The figure shows three views and two pictorial views of one solid part (mm, origin at its lowest corner). Answer the questions. A direction names the side the tool comes from. Coordinates: 2 decimals unless noted, no trailing zeros. Loops run counter-clockwise (first coordinate to the right, second up) from the corner with the lowest first, then second, coordinate; pieces in that order, holes last. Notation, with made-up numbers: (-39, -40) - (15, -40) arc R22 cw to (15, -33) - close; hole circle Ø4 at (33.25, 3.5). An arc over 180 degrees is marked (long way). One line per question, with ' | ' between items.
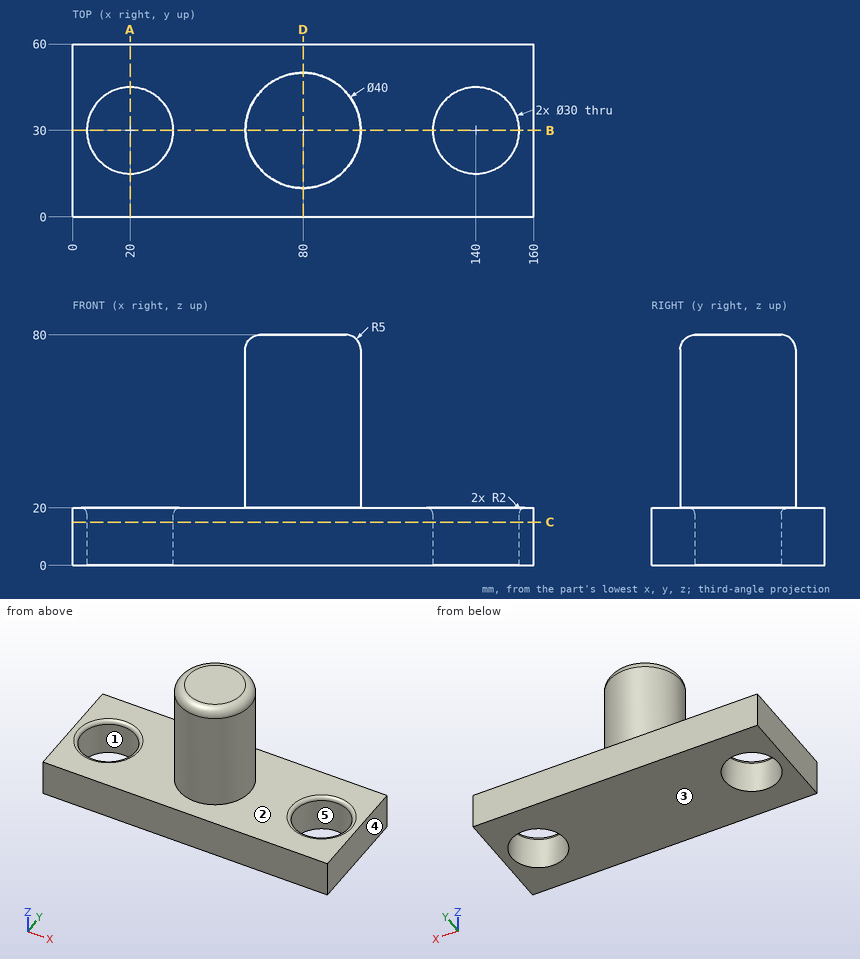
Item 1: Find the intervals of material crossed by line 1 (Y direction, x = 20, z = 8); line 2 (X direction, y = 27, z = 4.5); line 3 (Z direction, x = 8.5, y = 4), in increasing order. Write a range as [from, to].
Taken from the geometry:
line 1: y = [0, 15], [45, 60] | line 2: x = [0, 5.3], [34.7, 125.3], [154.7, 160] | line 3: z = [0, 20]
Item 2: Find section D-D, the plane x = 80. Write down the section's boundary in (y, z).
Taken from the geometry:
outline: (0, 0) - (60, 0) - (60, 20) - (50, 20) - (50, 75) arc R5 ccw to (45, 80) - (15, 80) arc R5 ccw to (10, 75) - (10, 20) - (0, 20) - close
Item 3: The mould has two halves that part along X. Classify the marked faces 3, 4 and 5: pulls with the +X half, pulls with the -X half, needs draft (parallel to the pull), parting line crosses it, or undercut.
Taken from the geometry:
face 3: needs draft | face 4: pulls with the +X half | face 5: undercut
Item 4: Which of the six approach directions +Z, -Z, +X, -X, +Y, -Y give full straight-line access (tool end or side, diameter ignored) to the marked faces 1 and 2?
Taken from the geometry:
face 1: +Z, -Z | face 2: +Z
Item 5: Find section A-A, the plane x = 20. Write down the section's boundary in (y, z).
Taken from the geometry:
outline: (0, 0) - (15, 0) - (15, 18) arc R2 ccw to (13, 20) - (0, 20) - close; (45, 0) - (60, 0) - (60, 20) - (47, 20) arc R2 ccw to (45, 18) - close
Item 6: Each of these flat-tipped pins is pushed along its axis until it touches: pin 1 Ø10 at (y, z) = (23.5, 63.5) entering from +X; pin 2 Ø8 at (x, z) = (84, 40.5) entering from -Y. Where does it stop, or does it pass through?
Taken from the geometry:
pin 1: stops at x = 99.94 | pin 2: stops at y = 10
Item 7: Find section C-C, the plane z = 15. Write down the section's boundary in (x, y).
Taken from the geometry:
outline: (0, 0) - (160, 0) - (160, 60) - (0, 60) - close; hole circle Ø30 at (20, 30); hole circle Ø30 at (140, 30)
Item 8: Find section B-B, the plane y = 30. Write down the section's boundary in (x, z), plus the area to 3 significant figures.
Taken from the geometry:
outline: (0, 0) - (5, 0) - (5, 18) arc R2 ccw to (3, 20) - (0, 20) - close; (35, 0) - (125, 0) - (125, 18) arc R2 ccw to (123, 20) - (100, 20) - (100, 75) arc R5 ccw to (95, 80) - (65, 80) arc R5 ccw to (60, 75) - (60, 20) - (37, 20) arc R2 ccw to (35, 18) - close; (155, 0) - (160, 0) - (160, 20) - (157, 20) arc R2 ccw to (155, 18) - close | area: 4,390 mm2
